```python
from build123d import *

# Parameters (mm, degrees)
F0_W     = 100
F0_H     = 100
F1_DEPTH = 14
F2_W     = 92
F2_H     = 90
F3_DEPTH = 12
F4_R     = 5


with BuildPart() as f1:
    # F0 (on Front) → F1 (new body)
    with BuildSketch(Plane.XZ):
        with Locations((5.404, 11.584203)):
            Rectangle(F0_W, F0_H)
    extrude(amount=F1_DEPTH)

    # F2 (on face) → F3 (cut)
    with BuildSketch(Plane.XZ.offset(14)):
        with Locations((6.02, 11.180203)):
            Rectangle(F2_W, F2_H)
    extrude(amount=-F3_DEPTH, mode=Mode.SUBTRACT)

    # F4
    f4_edges = [f1.edges().sort_by_distance(p)[0] for p in [
        (-44.596, -7, -38.415797),
        (55.404, -7, -38.415797),
        (55.404, -7, 61.584203),
        (-44.596, -7, 61.584203),
    ]]
    fillet(f4_edges, radius=F4_R)


solid = f1.part
```
Could you check a few things on this model? Use its own coordinates, in mm. A direction names the side the tool comes from. Coordinates: 2 decimals unless noted, no trailing zeros. Write each loop counter-clockwise with the first axis right and the second up, starting at its lowest first coordinate (ties: lowest second). Pieces come first, ordered by that corner, then holes. Notation, with made-up numbers: (-20.5, 57) -> (27.5, 57) arc R34 cw to (27.5, 93) -> close; hole circle Ø6 at (82, 38.5). An arc over 180 degrees is marked (long way). Return JSON: item names as keys, results as strings.
(1) Imagine slicing it at C-C, the plane z = 45.5. Please give me the cut outline in (x, y), then the cut area to 3 significant figures.
Numbers:
{"outline": "(-44.6, -14) -> (-39.98, -14) -> (-39.98, -2) -> (52.02, -2) -> (52.02, -14) -> (55.4, -14) -> (55.4, 0) -> (-44.6, 0) -> close", "area": "296 mm2"}
(2) Which directions (+Z, -Z, +X, -X, +Y, -Y) give clear straight access to the entire face, cutting with the end or side of a thin tool? Please do faces 5 (the flat face through (-44.596, -7, 11)), 6 (the flat face through (-39.98, -8, 11)).
Numbers:
{"face 5": "+Z, -Z, -X, +Y, -Y", "face 6": "-Y"}
(3) I'm going to push flat-ended pins straight in: pin 1 (1.5 mm diameter, centred on x = 32.5, z = 41, fed in from +Y); pin 2 (8 mm diameter, centred on x = -10.5, z = 13, fed in from -Y). Where does each tip first touch, or does it pass through?
Numbers:
{"pin 1": "stops at y = 0", "pin 2": "stops at y = -2"}
(4) I need wall thicknesses on L1, parallel to Z at x = 11, y = -3.5; L2, parallel to X at y = -5, z = 56; L3, parallel to Y at x = 39.5, z = 28.5. Which ranges of each line are inside material? Lowest first, please.
Numbers:
{"L1": "z = -38.42 to -33.82, 56.18 to 61.58", "L2": "x = -44.6 to -39.98, 52.02 to 55.4", "L3": "y = -2 to 0"}
(5) Imagine slicing it at A-A, the plane y = -5. Please give me the cut outline in (x, z).
Numbers:
{"outline": "(-44.6, -33.42) arc R5 ccw to (-39.6, -38.42) -> (50.4, -38.42) arc R5 ccw to (55.4, -33.42) -> (55.4, 56.58) arc R5 ccw to (50.4, 61.58) -> (-39.6, 61.58) arc R5 ccw to (-44.6, 56.58) -> close; hole (-39.98, -33.82) -> (52.02, -33.82) -> (52.02, 56.18) -> (-39.98, 56.18) -> close"}
(6) We'd pull the mould along Z, two halves only. Please class faces 1 (the flat face through (5, -8, -33.82)), 2 (the cylindrical face through (-43.17, -7.1, -36.91)), 3 (the cylindrical face through (-43.17, -7.1, 60.08)), 4 (the flat face through (5, 0, 12)): +Z half, -Z half, draft (parallel to the pull), parting line (faces both ways), or undercut.
Numbers:
{"face 1": "undercut", "face 2": "-Z half", "face 3": "+Z half", "face 4": "draft"}
(7) Imagine slicing it at B-B, the plane x = -2. Please give me the cut outline in (y, z).
Numbers:
{"outline": "(-14, -38.42) -> (0, -38.42) -> (0, 61.58) -> (-14, 61.58) -> (-14, 56.18) -> (-2, 56.18) -> (-2, -33.82) -> (-14, -33.82) -> close"}
